```python
from build123d import *


with BuildPart() as part:
    # 草图1 → 旋转2 (revolve)
    with BuildSketch(Plane.XY, mode=Mode.PRIVATE) as revolve_2_sk:
        with BuildLine():
            Line((-32, 15), (-37, 15))
            Line((-37, 15), (-37, 2))
            Line((-37, 2), (37, 2))
            Line((37, 2), (37, 15))
            Line((37, 15), (32, 15))
            ThreePointArc((32, 15), (30, 13), (28, 15))
            Line((28, 15), (-28, 15))
            ThreePointArc((-28, 15), (-30, 13), (-32, 15))
        make_face()
    revolve(revolve_2_sk.sketch.rotate(Axis((0, 0, 0), (1, 0, 0)), 90), axis=Axis((0, 0, 0), (1, 0, 0)))


solid = part.part
```
Geometry: final body of the model. Coordinates: model frame, mm. Round coordinates to 2 decimals unless told otherwise and drop trailing zeros. Write each loop counter-clockwise with the first axis right and the second up, starting at its lowest first coordinate (ties: lowest second). Pieces come first, ordered by that corner, then holes. Notation, with made-up numbers: M -39,51.5 L 3,51.5 A29 cw 3,86.5 Z; hole C -10,-26 d3. An arc over 180 degrees is marked long. Answer in a Markdown table with one row per item. Add a question column.
(1) Cut plane D-D, the plane x = 31. Return the cut outline in (y, z).
(2) Cut plane C-C, the plane x = -9. Return the cut outline in (y, z).
(3) Cut plane A-A, the plane z = 0. Return the cut outline in (x, y).
(4) Draft query along Z for faces 1 (the face through (-34.53, -12.65, 8.06)), 2 (the face through (1, 2, 0)), 3 (the face through (37, 0, -3)). Return one class per face: pulls with the +Z half, pulls with the -Z half, needs draft (parallel to the pull), parting line crosses it, or undercut.
(5) Contact query for flat-ended pins moving along their axis: pin 1 (2 mm diameter, centred on x = 11, z = 10, fed in from -Y); pin 2 (5 mm diameter, centred on x = -28, z = -8, fed in from +Y); pin 3 (2 mm diameter, centred on x = 12, z = 7.5, fed in from -Y); pin 4 (4 mm diameter, centred on x = -2.5, z = -1.5, fed in from +Y). Output: stop coordinate, or through.
(6) Ray query, L1, parallel to Y at x = -19, z = 0; L2, parallel to X at y = -4.5, z = 14; L3, parallel to X at y = -8.75, z = -11.5. Return the intervals inside material, ascending.
Established:
| question | item | result |
|---|---|---|
| 1 | outline | C 0,0 d26.54; hole C 0,0 d4 |
| 2 | outline | C 0,0 d30; hole C 0,0 d4 |
| 3 | outline | M -37,-15 L -32,-15 A2 cw -28,-15 L 28,-15 A2 cw 32,-15 L 37,-15 L 37,-2 L -37,-2 Z; M -37,2 L 37,2 L 37,15 L 32,15 A2 cw 28,15 L -28,15 A2 cw -32,15 L -37,15 Z |
| 4 | face 1 | parting line crosses it |
| 4 | face 2 | undercut |
| 4 | face 3 | needs draft |
| 5 | pin 1 | y = -12 |
| 5 | pin 2 | y = 13.96 |
| 5 | pin 3 | y = -13.52 |
| 5 | pin 4 | y = 15 |
| 6 | L1 | -15 to -2, 2 to 15 |
| 6 | L2 | -37 to -31.98, -28.02 to 28.02, 31.98 to 37 |
| 6 | L3 | -37 to -31.92, -28.08 to 28.08, 31.92 to 37 |
